```python
from build123d import *

# Parameters (mm, degrees)
SKETCH1_W           = 58
SKETCH1_H           = 10
SKETCH1_R           = 2
BOSS_EXTRUDE1_DEPTH = 55
SKETCH3_W           = 58
SKETCH3_H           = 10
CUT_EXTRUDE3_DEPTH  = 10
SKETCH4_R           = 5
CUT_EXTRUDE4_DEPTH  = 10


with BuildPart() as part:
    # Sketch1 → Boss-Extrude1 (new body)
    with BuildSketch(Plane.XY):
        with Locations((29, -5)):
            Rectangle(SKETCH1_W, SKETCH1_H)
        with Locations((14, -5)):
            Circle(SKETCH1_R, mode=Mode.SUBTRACT)
        with Locations((44, -5)):
            Circle(SKETCH1_R, mode=Mode.SUBTRACT)
    extrude(amount=BOSS_EXTRUDE1_DEPTH)

    # Sketch3 → Cut-Extrude3 (cut)
    with BuildSketch(Plane(origin=(0, 0, 0), x_dir=(-1, 0, 0), z_dir=(0, 0, -1))):
        with Locations((-29, -5)):
            Rectangle(SKETCH3_W, SKETCH3_H)
    extrude(amount=-CUT_EXTRUDE3_DEPTH, mode=Mode.SUBTRACT)

    # Sketch4 → Cut-Extrude4 (cut)
    with BuildSketch(Plane(origin=(0, 0, 0), x_dir=(1, 0, 0), z_dir=(0, 1, 0))):
        with Locations(Location((29, -21.5, 0), (0, 0, 270))):
            Circle(SKETCH4_R)
    extrude(amount=-CUT_EXTRUDE4_DEPTH, mode=Mode.SUBTRACT)


solid = part.part
```
Verification items for the finished model (mm, model axes). Give positions to 0.01 mm unless a question says otherwise; leave off trailing zeros. Order: outer loops, then holes, each group sorted by start corner. A loop starts at its lowest first (then second) coordinate and runs counter-clockwise, first axis right, second up. Notation, with made-up numbers: M 35.25,38 L 83.25,38 A30 cw 83.25,73 Z; hole C 35,-29.5 d3. An arc over 180 degrees is marked long. Answer in a Markdown table with one row per item. Add a question column.
Item 1: Section check B-B, the plane y = -5. Enter the section's corners in (x, z).
Item 2: Mould release check, pull along Y, two halves, no side actions. Record for faces 1 (the flat face through (29, -5, 55)), 2 (the flat face through (29, -10, 32)), 3 (the cylindrical face through (12.4, -6.2, 32.2)): released by +Y, released by -Y, zero draft, split by the parting line, or undercut.
Item 3: Section check D-D, the plane z = 48.5. Enter the section's corners in (x, y).
Item 4: Section check A-A, the plane z = 21.5. Enter the section's corners in (x, y).
Item 5: Gauge pin test, flat end, axial feed: pin 1 (6 mm diameter, centred on x = 29, z = 21.5, fed in from +Y). Record the tip position at first contact, or that the pin passes through.
Item 6: Section check C-C, the plane x = 44. Enter the section's corners in (y, z).
Item 7: Scan lines: probe 1 along X at (y, z) = (-5, 30); probe 2 along Y at (x, z) = (44, 19); probe 3 along X at (y, z) = (-3.5, 34). Record each from-to range of solid material in increasing order. Write a range as from..to.
Filled sheet:
| question | item | result |
|---|---|---|
| 1 | outline | M 0,10 L 12,10 L 12,55 L 0,55 Z; M 16,10 L 42,10 L 42,55 L 16,55 Z; M 46,10 L 58,10 L 58,55 L 46,55 Z; hole C 29,21.5 d10 |
| 2 | face 1 | zero draft |
| 2 | face 2 | released by -Y |
| 2 | face 3 | undercut |
| 3 | outline | M 0,-10 L 58,-10 L 58,0 L 0,0 Z; hole C 14,-5 d4; hole C 44,-5 d4 |
| 4 | outline | M 0,-10 L 24,-10 L 24,0 L 0,0 Z; M 34,-10 L 58,-10 L 58,0 L 34,0 Z; hole C 14,-5 d4; hole C 44,-5 d4 |
| 5 | pin 1 | passes through |
| 6 | outline | M -10,10 L -7,10 L -7,55 L -10,55 Z; M -3,10 L 0,10 L 0,55 L -3,55 Z |
| 7 | probe 1 | x = 0..12, 16..42, 46..58 |
| 7 | probe 2 | y = -10..-7, -3..0 |
| 7 | probe 3 | x = 0..12.68, 15.32..42.68, 45.32..58 |
